Can you work these out from the drawing? Everything is in mm from the part's minimum corner. Give positions to 0.01 mm unless a question says otherwise; leave off trailing zeros. Write each loop counter-clockwise with the first axis right and the second up, starting at its lowest first coordinate (ties: lowest second). Pieces come first, ordered by that corner, then holes. Notation, with made-up numbers: (80, -31) - (95, -31) arc R12 ccw to (95, -27) - close; hole circle Ø1 at (-8, 66.25). An arc over 180 degrees is marked (long way). Use a Markdown table: item, result.
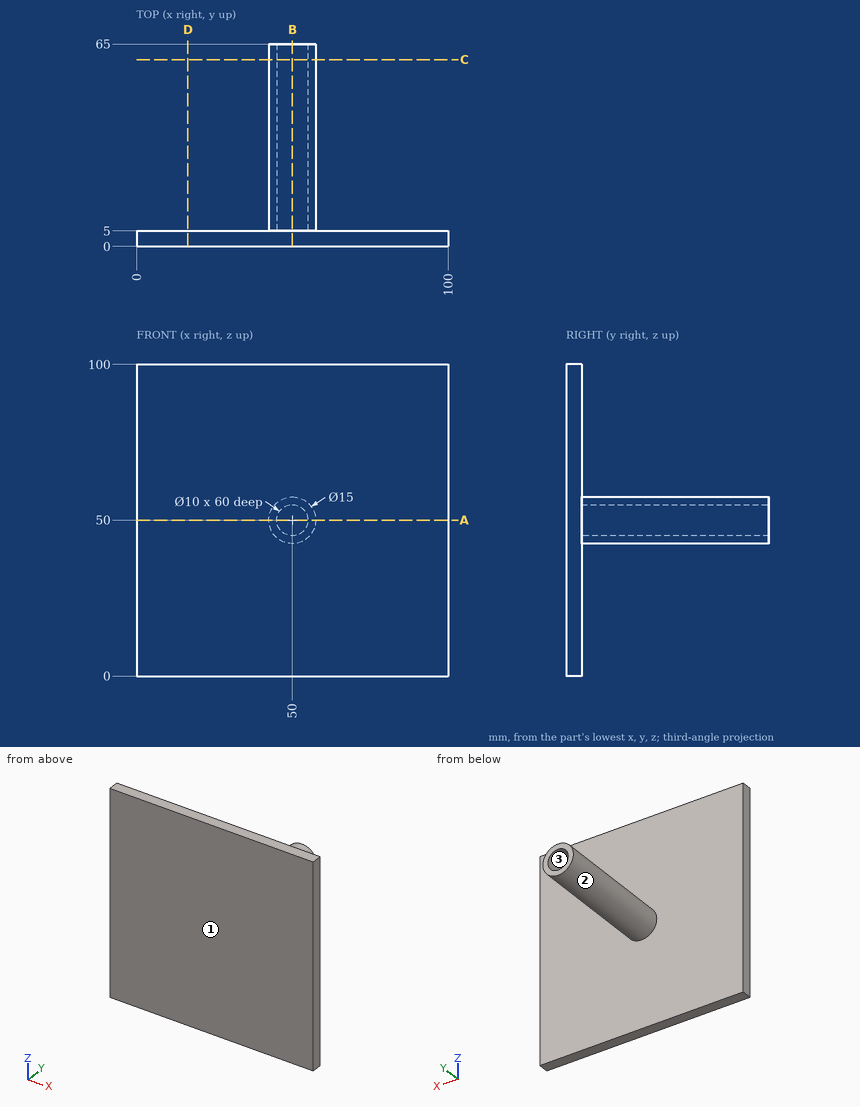
Item 1: I need wall thicknesses on line 1 along X through (y, z) = (29.5, 50); line 2 along Y through (x, z) = (6, 5); line 3 along Z through (x, y) = (43.5, 48.5). Which ranges of each line are inside material? Lowest first, please. Write a range as [from, to].
Values:
| item | result |
|---|---|
| line 1 | x = [42.5, 45], [55, 57.5] |
| line 2 | y = [0, 5] |
| line 3 | z = [46.26, 53.74] |
Item 2: If we section it at D-D, the plane x = 16.5: Write out the boundary of the cut face in (y, z), plus the area to 3 significant figures.
Values:
| item | result |
|---|---|
| outline | (0, 0) - (5, 0) - (5, 100) - (0, 100) - close |
| area | 500 mm2 |
Item 3: Thinking about a two-plate mould opening in X: for the marked faces 1, 2 and 3, which applies, +X half, -X half, draft (parallel to the pull), parting line (faces both ways), or undercut?
Values:
| item | result |
|---|---|
| face 1 | draft |
| face 2 | parting line |
| face 3 | undercut |
Item 4: If we section it at B-B, the plane x = 50: Write out the boundary of the cut face in (y, z).
Values:
| item | result |
|---|---|
| outline | (0, 0) - (5, 0) - (5, 42.5) - (65, 42.5) - (65, 45) - (5, 45) - (5, 55) - (65, 55) - (65, 57.5) - (5, 57.5) - (5, 100) - (0, 100) - close |
Item 5: If we section it at C-C, the plane y = 60: Write out the boundary of the cut face in (x, z), plus the area to 3 significant figures.
Values:
| item | result |
|---|---|
| outline | circle Ø15 at (50, 50); hole circle Ø10 at (50, 50) |
| area | 98.2 mm2 |
Item 6: If we section it at A-A, the plane z = 50: Write out the boundary of the cut face in (x, y).
Values:
| item | result |
|---|---|
| outline | (0, 0) - (100, 0) - (100, 5) - (57.5, 5) - (57.5, 65) - (55, 65) - (55, 5) - (45, 5) - (45, 65) - (42.5, 65) - (42.5, 5) - (0, 5) - close |
Item 7: Will these pins go through, and if not, where does the flat tip stop? pin 1 Ø12 at (x, y) = (58, 33.5) entering from +Z; pin 2 Ø1 at (x, z) = (56.5, 79) entering from -Y; pin 3 Ø8 at (x, z) = (74.5, 46.5) entering from +Y.
Values:
| item | result |
|---|---|
| pin 1 | stops at z = 57.23 |
| pin 2 | stops at y = 0 |
| pin 3 | stops at y = 5 |
